For this review, take the finished solid that the model builds, in its own axes (mm). A direction names the side the tool comes from. Give positions to 0.01 mm unless a question says otherwise; leave off trailing zeros. Order: outer loops, then holes, each group sorted by start corner. A loop starts at its lowest first (then second) coordinate and runs counter-clockwise, first axis right, second up. Notation, with made-up numbers: (23.5, 85.5) - (79.5, 85.5) arc R14 ccw to (79.5, 108.5) - close; hole circle Ø7 at (46.5, 1). An arc over 180 degrees is marked (long way). One line per item, written item: value.
```python
from build123d import *

# Parameters (mm, degrees)
SKETCH1_R                = 323.85
BOSS_EXTRUDE3_DEPTH      = 101.6
BOSS_EXTRUDE4_DEPTH      = 25.4
BOSS_EXTRUDE4_DEPTH_BACK = 127
SKETCH2_R                = 114.3
BOSS_EXTRUDE5_DEPTH      = 38.1
BOSS_EXTRUDE5_DEPTH_BACK = 190.5
SKETCH4_R                = 88.9
BOSS_EXTRUDE6_DEPTH      = 184.15
BOSS_EXTRUDE6_DEPTH_BACK = 412.75
SKETCH5_R                = 44.45
BOSS_EXTRUDE7_DEPTH      = 50.8
BOSS_EXTRUDE7_DEPTH_BACK = 25.4
SKETCH6_R                = 12.7
FILLET2_R                = 12.7


with BuildPart() as part:
    # Sketch1 → Boss-Extrude3 (new body)
    with BuildSketch(Plane.XY):
        Circle(SKETCH1_R)
    extrude(amount=BOSS_EXTRUDE3_DEPTH)

    # Sketch2 → Boss-Extrude4 (add, two sides: drawn at the far end of the back side and taken through both)
    with BuildSketch(Plane.XY.offset(101.6).offset(-BOSS_EXTRUDE4_DEPTH_BACK)):
        Circle(SKETCH2_R)
    extrude(amount=BOSS_EXTRUDE4_DEPTH + BOSS_EXTRUDE4_DEPTH_BACK)

    # Sketch4 → Boss-Extrude5 (add, two sides: drawn at the far end of the back side and taken through both)
    with BuildSketch(Plane.XY.offset(127).offset(-BOSS_EXTRUDE5_DEPTH_BACK)):
        Circle(SKETCH4_R)
    extrude(amount=BOSS_EXTRUDE5_DEPTH + BOSS_EXTRUDE5_DEPTH_BACK)

    # Sketch5 → Boss-Extrude6 (add, two sides: drawn at the far end of the back side and taken through both)
    with BuildSketch(Plane.XY.offset(165.1).offset(-BOSS_EXTRUDE6_DEPTH_BACK)):
        Circle(SKETCH5_R)
    extrude(amount=BOSS_EXTRUDE6_DEPTH + BOSS_EXTRUDE6_DEPTH_BACK)

    # Sketch6 → Boss-Extrude7 (add, two sides: drawn at the far end of the back side and taken through both)
    with BuildSketch(Plane(origin=(0, 44.45, 0), x_dir=(1, 0, 0), z_dir=(0, 1, 0)).offset(-BOSS_EXTRUDE7_DEPTH_BACK)):
        with Locations(Location((0, -317.5, 0), (0, 0, 270))):
            Circle(SKETCH6_R)
    extrude(amount=BOSS_EXTRUDE7_DEPTH + BOSS_EXTRUDE7_DEPTH_BACK)

    # Fillet2
    fillet2_edges = [part.edges().sort_by_distance(p)[0] for p in [
        (0, 95.25, 304.8),
    ]]
    fillet(fillet2_edges, radius=FILLET2_R)


solid = part.part
```
(1) Wall thickness on line 1 (Z direction, x = -141.5, y = 70.5); line 2 (Z direction, x = 49, y = -100); line 3 (Y direction, x = 283.5, z = 41): over which ranges is each line inside the solid? List them lowest first. Write a range as from..to.
Answers below:
line 1: z = 0..101.6
line 2: z = -25.4..127
line 3: y = -156.55..156.55
(2) Take a section at D-D (x = -100.5). Write out the cut boundary in (y, z).
Answers below:
outline: (-307.86, 0) - (-54.44, 0) - (-54.44, -25.4) - (54.44, -25.4) - (54.44, 0) - (307.86, 0) - (307.86, 101.6) - (54.44, 101.6) - (54.44, 127) - (-54.44, 127) - (-54.44, 101.6) - (-307.86, 101.6) - close
(3) Take a section at B-B (y = 0). Write out the cut boundary in (x, z), then the cut area to 3 significant figures.
Answers below:
outline: (-323.85, 0) - (-114.3, 0) - (-114.3, -25.4) - (-88.9, -25.4) - (-88.9, -63.5) - (-44.45, -63.5) - (-44.45, -247.65) - (44.45, -247.65) - (44.45, -63.5) - (88.9, -63.5) - (88.9, -25.4) - (114.3, -25.4) - (114.3, 0) - (323.85, 0) - (323.85, 101.6) - (114.3, 101.6) - (114.3, 127) - (88.9, 127) - (88.9, 165.1) - (44.45, 165.1) - (44.45, 349.25) - (-44.45, 349.25) - (-44.45, 165.1) - (-88.9, 165.1) - (-88.9, 127) - (-114.3, 127) - (-114.3, 101.6) - (-323.85, 101.6) - close
area: 124,000 mm^2
(4) Take a section at C-C (z = -43.5). Write out the cut boundary in (x, y), then the cut area to 3 significant figures.
Answers below:
outline: circle Ø177.8 at (0, 0)
area: 24,800 mm^2
(5) For P1, Ø1, axis at x = 143.5, z = 90.5, coming from the -Y side; P2, Ø12, axis at x = 44.5, z = 228.5, coming from the +Y side; P3, Ø8, axis at y = 24.5, z = -96, coming from the +X side, all flat-tipped, find the tip position at first contact; note any pin that passes through.
Answers below:
P1: stops at y = -290.57
P2: stops at y = 22.22
P3: stops at x = 39.44
(6) Draft analysis for pull direction Z (two halves, no side actions). For faces 1 (the face through (-42.159, 321.094, 50.089)), 2 (the face through (3.815, 62.293, 329.614)), 3 (the face through (-1, 1, -247.65)), 4 (the face through (-1, 1, 349.25)), state which applies: pulls with the +Z half, pulls with the -Z half, needs draft (parallel to the pull), parting line crosses it, or undercut.
Answers below:
face 1: needs draft
face 2: undercut
face 3: pulls with the -Z half
face 4: pulls with the +Z half
(7) Machinability: for faces 5 (the face through (139, 5, 101.6)), 6 (the face through (139, 5, 0)), which of the approach directions +Z, -Z, +X, -X, +Y, -Y give a long, thin tool a straight path to every point of the face, cutting with its end or side? Answer none if there is none.
Answers below:
face 5: +Z
face 6: -Z
